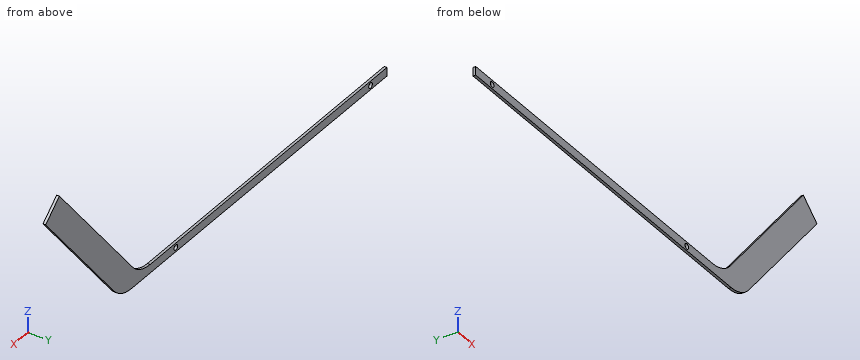
```python
from build123d import *

# Parameters (mm, degrees)
F1_DEPTH = 4
F2_R     = 4
F3_DEPTH = 25


with BuildPart() as f1:
    # F0 (on Front) → F1 (new body)
    with BuildSketch(Plane.XZ):
        with BuildLine():
            Line((-219.300896, 13), (-219.300896, 0))
            Line((-219.300896, 0), (343.669184, 0))
            ThreePointArc((343.669184, 0), (365.194739, 4.870736), (382.526482, 18.53398))
            Line((382.526482, 18.53398), (532.675548, 203.952635))
            Line((532.675548, 203.952635), (502.477538, 230.221827))
            Line((502.477538, 230.221827), (341.583292, 31.53398))
            ThreePointArc((341.583292, 31.53398), (324.251549, 17.870736), (302.725994, 13))
            Line((302.725994, 13), (-219.300896, 13))
        make_face()
    extrude(amount=F1_DEPTH)

    # F2 (on face) → F3 (cut)
    with BuildSketch(Plane.XZ.offset(4)):
        with Locations((245.786324, 6.5)):
            Circle(F2_R)
        with Locations((-182.988614, 6.5)):
            Circle(F2_R)
    extrude(amount=-F3_DEPTH, mode=Mode.SUBTRACT)


solid = f1.part
```
Here's how the part is built. I have some questions about the finished solid (model axes, mm). Give positions to 0.01 mm unless a question says otherwise; leave off trailing zeros. Loops run counter-clockwise (first coordinate to the right, second up) from the corner with the lowest first, then second, coordinate; pieces in that order, holes last. Notation, with made-up numbers: (77.25, 48.25) -> (104.25, 48.25) arc R16 ccw to (104.25, 52.25) -> close; hole circle Ø3 at (59.5, 77.5). An arc over 180 degrees is marked (long way). Use one line per item in the form item = value. Start each with the question number.
1) Please list where these lines run through material, in increasing order: line 1 along Z through (x, y) = (-42, -3.05); line 2 along Z through (x, y) = (-184, -2); line 3 along Z through (x, y) = (-186, -0.4).
2) Imagine slicing it at C-C (z = 87). Please give me the cut outline in (x, y).
3) Imagine slicing it at A-A (y = -1.95). Please give me the cut outline in (x, z).
4) For P1, Ø2, axis at y = -3, z = 30.5, coming from the -X side; P2, Ø2, axis at x = 148, y = -1.5, coming from the +Z side; P3, Ø9, axis at x = -182.99, z = 6.5, coming from the -Y side, each with a flat end and sliding along its axis, tell me the tip position at first contact or that it passes through.
5) Imagine slicing it at B-B (x = -163). Please give me the cut outline in (y, z).
Check values:
q1.line_1 = 0 to 13
q1.line_2 = 0 to 2.63, 10.37 to 13
q1.line_3 = 0 to 3.87, 9.13 to 13
q2.outline = (386.5, -4) -> (437.97, -4) -> (437.97, 0) -> (386.5, 0) -> close
q3.outline = (-219.3, 0) -> (343.67, 0) arc R50 ccw to (382.53, 18.53) -> (532.68, 203.95) -> (502.48, 230.22) -> (341.58, 31.53) arc R50 cw to (302.73, 13) -> (-219.3, 13) -> close; hole circle Ø8 at (-182.99, 6.5); hole circle Ø8 at (245.79, 6.5)
q4.P1 = 339.84
q4.P2 = 13
q4.P3 = -4
q5.outline = (-4, 0) -> (0, 0) -> (0, 13) -> (-4, 13) -> close
